The listing builds one solid part. Answer for the finished solid, in the listing's coordinates (mm). A direction names the side the tool comes from. Coordinates: 2 decimals unless noted, no trailing zeros. Write each loop counter-clockwise with the first axis right and the second up, starting at its lowest first coordinate (ties: lowest second). Pieces come first, ordered by that corner, then holes.
(1) The part is cut by section A-A on z = 8. Determine the outline of the cut face in (x, y), plus the area to 3 significant figures.
(2) Given P1, Ø5, axis at x = -9, z = -13.5, coming from the +Y side; P2, Ø6, axis at x = 4, y = 25.5, coming from the -Z side, each flat-ended and moving along its own axis, determine where each tip first touches the part or whether it passes through.
(3) The part is cut by section B-B on x = 11. Determine the outline of the cut face in (y, z).
(4) Which of the six approach directions +Z, -Z, +X, -X, +Y, -Y give full straight-line access (tool end or side, diameter ignored) to faces 1 (the flat face through (0, 10, -20)), 2 (the flat face through (-10, 30, 5)), 3 (the flat face through (10, 30, -10))?
(5) The part is cut by section D-D on y = 29. Determine the outline of the cut face in (x, z), plus the area to 3 significant figures.
(6) Straight lines are drawn through the part: line 1 (Y direction, x = -19, z = -14); line 2 (Z direction, x = 13, y = 22.5); line 3 (X direction, y = 25.5, z = -6.5). For each, find the intervals that lie inside material, in ascending order.
(7) The part is cut by section C-C on y = 21. Determine the outline of the cut face in (x, z).
from build123d import *

# Parameters (mm, degrees)
CROQUIS1_W              = 60
CROQUIS1_H              = 40
SALIENTE_EXTRUIR2_DEPTH = 20
CROQUIS3_W              = 40
CROQUIS3_H              = 30
SALIENTE_EXTRUIR3_DEPTH = 20
CHAFL_N1_START          = 40.529988897
CHAFL_N1_OUTLINE_W      = 28
CHAFL_N1_OUTLINE_H      = 31
CHAFL_N1_DEPTH          = 12.470011103


with BuildPart() as part:
    # Croquis1 → Saliente-Extruir2 (new body)
    with BuildSketch(Plane(origin=(0, 0, 0), x_dir=(1, 0, 0), z_dir=(0, 1, 0))):
        Rectangle(CROQUIS1_W, CROQUIS1_H)
    extrude(amount=SALIENTE_EXTRUIR2_DEPTH)

    # Croquis3 → Saliente-Extruir3 (add)
    with BuildSketch(Plane(origin=(0, 20, 0), x_dir=(1, 0, 0), z_dir=(0, 1, 0))):
        with Locations((10, -5)):
            Rectangle(CROQUIS3_W, CROQUIS3_H)
    extrude(amount=SALIENTE_EXTRUIR3_DEPTH)

    # Chaflán1: read off the stored shape, not the designer's step
    # Chaflán1 outline → Chaflán1 (cut)
    with BuildSketch(Plane(origin=(0, 0, 0), x_dir=(0.8164965809277258, -0.40824829046386313, -0.40824829046386313), z_dir=(0.5773502691896258, 0.5773502691896258, 0.5773502691896258)).offset(CHAFL_N1_START)):
        with Locations((-4, 14.5)):
            Rectangle(CHAFL_N1_OUTLINE_W, CHAFL_N1_OUTLINE_H)
    extrude(amount=CHAFL_N1_DEPTH, mode=Mode.SUBTRACT)


solid = part.part
Model answer:
1. outline: (-30, 0) - (30, 0) - (30, 32.2) - (22.2, 40) - (-10, 40) - (-10, 20) - (-30, 20) - close
1. area: 1,970 mm2
2. P1: stops at y = 20
2. P2: stops at z = -10
3. outline: (0, -20) - (20, -20) - (20, -10) - (40, -10) - (40, 19.2) - (39.2, 20) - (0, 20) - close
4. face 1: -Z, +X, -X, +Y, -Y
4. face 2: +Z, -Z, -X, +Y
4. face 3: -Z, +X, -X, +Y
5. outline: (-10, -10) - (30, -10) - (30, 11.2) - (21.2, 20) - (-10, 20) - close
5. area: 1,160 mm2
6. line 1: y = 0 to 20
6. line 2: z = -10 to 20
6. line 3: x = -10 to 30
7. outline: (-10, -10) - (30, -10) - (30, 19.2) - (29.2, 20) - (-10, 20) - close
